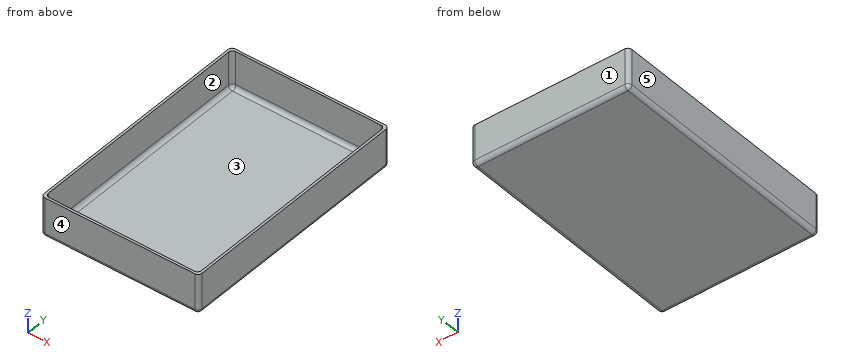
```python
from build123d import *

# Parameters (mm, degrees)
F0_W     = 80
F0_H     = 120
F1_DEPTH = 20
F2_W     = 77.6
F2_H     = 117.6
F3_DEPTH = 18.8
F4_R     = 2
F5_R     = 2
F6_R     = 2
F7_R     = 2


with BuildPart() as f1:
    # F0 (on Top) → F1 (new body)
    with BuildSketch(Plane.XY):
        Rectangle(F0_W, F0_H)
    extrude(amount=F1_DEPTH)

    # F2 (on face) → F3 (cut)
    with BuildSketch(Plane.XY.offset(20)):
        Rectangle(F2_W, F2_H)
    extrude(amount=-F3_DEPTH, mode=Mode.SUBTRACT)

    # F4
    f4_edges = [f1.edges().sort_by_distance(p)[0] for p in [
        (40, -60, 10),
        (40, 60, 10),
        (-40, -60, 10),
        (-40, 60, 10),
    ]]
    fillet(f4_edges, radius=F4_R)

    # F5
    f5_edges = [f1.edges().sort_by_distance(p)[0] for p in [
        (-38.8, 58.8, 10.6),
        (-38.8, -58.8, 10.6),
        (38.8, -58.8, 10.6),
        (38.8, 58.8, 10.6),
    ]]
    fillet(f5_edges, radius=F5_R)

    # F6
    f6_edges = [f1.edges().sort_by_distance(p)[0] for p in [
        (0, -58.8, 1.2),
        (-38.214214, -58.214214, 1.2),
        (38.214214, -58.214214, 1.2),
        (-38.8, 0, 1.2),
        (38.8, 0, 1.2),
        (-38.214214, 58.214214, 1.2),
        (38.214214, 58.214214, 1.2),
        (0, 58.8, 1.2),
    ]]
    fillet(f6_edges, radius=F6_R)

    # F7
    f7_edges = [f1.edges().sort_by_distance(p)[0] for p in [
        (-40, 0, 0),
        (-39.414214, 59.414214, 0),
        (-39.414214, -59.414214, 0),
        (0, 60, 0),
        (0, -60, 0),
        (39.414214, 59.414214, 0),
        (39.414214, -59.414214, 0),
        (40, 0, 0),
    ]]
    fillet(f7_edges, radius=F7_R)


solid = f1.part
```
Read the model definition and answer for the solid it produces. Units are mm, in the model's axes. Face numbers are marked on the shaded views. A direction names the side the tool comes from. Round coordinates to 2 decimals unless told otherwise and drop trailing zeros. Loops run counter-clockwise (first coordinate to the right, second up) from the corner with the lowest first, then second, coordinate; pieces in that order, holes last. Notation, with made-up numbers: (45.5, 24) -> (75.5, 24) arc R21 ccw to (75.5, 36) -> close; hole circle Ø9 at (85.25, 29). An arc over 180 degrees is marked (long way). One line per item, written item: value.
1) A flat-ended cylindrical pin translates along its axis: P1, Ø1.5, axis at x = -5, y = -45.5, coming from the +Z side. Find the tip coordinate at first contact, or state that the pin passes through.
Answer list:
P1: stops at z = 1.2
2) A cutting plane is placed at A-A (x = -16). Determine the outline of the cut face in (y, z), and give its area (3 significant figures).
Answer list:
outline: (-60, 2) arc R2 ccw to (-58, 0) -> (58, 0) arc R2 ccw to (60, 2) -> (60, 20) -> (58.8, 20) -> (58.8, 3.2) arc R2 cw to (56.8, 1.2) -> (-56.8, 1.2) arc R2 cw to (-58.8, 3.2) -> (-58.8, 20) -> (-60, 20) -> close
area: 189 mm²
3) For the marked faces 1 and 2, determine the directions among +Z, -Z, +X, -X, +Y, -Y from which every point of the face is accessible in a straight line to the end or side of a thin tool.
Answer list:
face 1: +Z, -Z, +X, -X, +Y
face 2: +Z
4) A cutting plane is placed at B-B (z = 8.25). Determine the outline of the cut face in (x, y).
Answer list:
outline: (-40, -58) arc R2 ccw to (-38, -60) -> (38, -60) arc R2 ccw to (40, -58) -> (40, 58) arc R2 ccw to (38, 60) -> (-38, 60) arc R2 ccw to (-40, 58) -> close; hole (-38.8, -56.8) arc R2 ccw to (-36.8, -58.8) -> (36.8, -58.8) arc R2 ccw to (38.8, -56.8) -> (38.8, 56.8) arc R2 ccw to (36.8, 58.8) -> (-36.8, 58.8) arc R2 ccw to (-38.8, 56.8) -> close
5) Consider L1, parallel to X at y = 41.5, z = 9.5; L2, parallel to Y at x = -31, z = 14; L3, parallel to Z at x = -21, y = -37. Determine where each line is inside the solid, lowest interval first. Write a range as [from, to].
Answer list:
L1: x = [-40, -38.8], [38.8, 40]
L2: y = [-60, -58.8], [58.8, 60]
L3: z = [0, 1.2]
6) The mould has two halves that part along X. Classify the marked faces 3, 4 and 5: pulls with the +X half, pulls with the -X half, needs draft (parallel to the pull), parting line crosses it, or undercut.
Answer list:
face 3: undercut
face 4: needs draft
face 5: pulls with the -X half
7) A cutting plane is placed at C-C (y = 46). Determine the outline of the cut face in (x, z).
Answer list:
outline: (-40, 2) arc R2 ccw to (-38, 0) -> (38, 0) arc R2 ccw to (40, 2) -> (40, 20) -> (38.8, 20) -> (38.8, 3.2) arc R2 cw to (36.8, 1.2) -> (-36.8, 1.2) arc R2 cw to (-38.8, 3.2) -> (-38.8, 20) -> (-40, 20) -> close
